Verification items for the finished model (mm, model axes). Round coordinates to 2 decimals unless told otherwise and drop trailing zeros. Write each loop counter-clockwise with the first axis right and the second up, starting at its lowest first coordinate (ties: lowest second). Pieces come first, ordered by that corner, then holes. Notation, with made-up numbers: (-10, 41) -> (15, 41) arc R20 cw to (15, 76) -> close; hole circle Ø6 at (25.25, -31). An arc over 180 degrees is marked (long way). Answer as a JSON object with one key per item and string values. Group by question number.
(1) Gauge pin test, flat end, axial feed: pin 1 Ø1.5 at (x, z) = (4.375, -5) entering from -Y. Record the tip position at first contact, or that the pin passes through.
(2) Scan lines: L1, parallel to X at y = 0.25, z = -168 (3 decimals); L2, parallel to X at y = 0.3, z = -37.5 (3 decimals); L3, parallel to Z at x = 3.5, y = 0.15. Record each from-to range of solid material in increasing order. Write a range as from..to.
(3) Sectioned sample at B-B on z = -103.5. Record the cut outline in (x, y) (3 decimals).
(4) Sectioned sample at A-A on y = 0.4. Count the separate pieces of the cut face and the enclosed holes in it, and give its area (3 significant figures).
```python
from build123d import *

# Parameters (mm, degrees)
SKETCH4_R           = 1.5
SKETCH4_R_2         = 1.25
BOSS_EXTRUDE2_DEPTH = 0.5


with BuildPart() as part:
    # Sketch4 → Boss-Extrude2 (new body)
    with BuildSketch(Plane(origin=(0, 0, 0), x_dir=(1, 0, 0), z_dir=(0, 1, 0))):
        with BuildLine():
            Line((0, 128.6), (0, 0))
            Line((0, 0), (-65.208953904, 0))
            ThreePointArc((-65.208953904, 0), (-75.225861161, 4.149138839), (-79.375, 14.166046096))
            Line((-79.375, 14.166046096), (-79.375, 50))
            Line((-79.375, 50), (-49.375, 50))
            Line((-49.375, 50), (-49.375, 118))
            Line((-49.375, 118), (-64.675, 118))
            ThreePointArc((-64.675, 118), (-75.069469683, 122.305530317), (-79.375, 132.7))
            Line((-79.375, 132.7), (-79.375, 193.786049975))
            add(Edge.make_bspline(
                [(-79.375, 193.786049975), (-78.783979858, 199.964089634), (-73.952599984, 211.643726286), (-54.660456042, 223.601842558), (-29.545703417, 228.182905558), (-9.188135392, 228.171492971), (0, 228.6)],
                knots=[0, 0, 0, 0, 0.226113446, 0.328670148, 0.719907193, 1, 1, 1, 1], degree=3))
            Line((0, 228.6), (0, 188.6))
            Line((0, 188.6), (-50, 188.6))
            ThreePointArc((-50, 188.6), (-51.25, 187.35), (-50, 186.1))
            Line((-50, 186.1), (0, 186.1))
            Line((0, 186.1), (0, 179.6))
            Line((0, 179.6), (-50, 179.6))
            ThreePointArc((-50, 179.6), (-51.25, 178.35), (-50, 177.1))
            Line((-50, 177.1), (0, 177.1))
            Line((0, 177.1), (0, 131.1))
            Line((0, 131.1), (-50, 131.1))
            ThreePointArc((-50, 131.1), (-51.25, 129.85), (-50, 128.6))
            Line((-50, 128.6), (0, 128.6))
        make_face()
        with Locations(Location((-74.875, 43, 0), (0, 0, 270))):
            Circle(SKETCH4_R, mode=Mode.SUBTRACT)
        with Locations(Location((-74.875, 18, 0), (0, 0, 270))):
            Circle(SKETCH4_R, mode=Mode.SUBTRACT)
        with Locations(Location((-39.375, 7.5, 0), (0, 0, 270))):
            Circle(SKETCH4_R, mode=Mode.SUBTRACT)
        with Locations(Location((-13.375, 7.5, 0), (0, 0, 270))):
            Circle(SKETCH4_R, mode=Mode.SUBTRACT)
        with Locations(Location((-4.375, 5, 0), (0, 0, 270))):
            Circle(SKETCH4_R_2, mode=Mode.SUBTRACT)
        with Locations(Location((-74.375, 143, 0), (0, 0, 270))):
            Circle(SKETCH4_R, mode=Mode.SUBTRACT)
        with Locations(Location((-74.375, 168, 0), (0, 0, 270))):
            Circle(SKETCH4_R, mode=Mode.SUBTRACT)
        with Locations(Location((-74.375, 193, 0), (0, 0, 270))):
            Circle(SKETCH4_R, mode=Mode.SUBTRACT)
        with Locations(Location((-39.375, 37.5, 0), (0, 0, 270))):
            Circle(SKETCH4_R, mode=Mode.SUBTRACT)
        with Locations(Location((-39.375, 67.5, 0), (0, 0, 270))):
            Circle(SKETCH4_R, mode=Mode.SUBTRACT)
        with Locations(Location((-12.875, 37.5, 0), (0, 0, 270))):
            Circle(SKETCH4_R, mode=Mode.SUBTRACT)
        with Locations(Location((-12.875, 67.5, 0), (0, 0, 270))):
            Circle(SKETCH4_R, mode=Mode.SUBTRACT)
    boss_extrude2 = extrude(amount=BOSS_EXTRUDE2_DEPTH)

    # Mirror4: part across plane


with BuildPart() as part_1:
    add(part.part)
    add(part.part.mirror(Plane(origin=(0, 0.5, -177.1), x_dir=(0, 0, 1), z_dir=(-1, 0, 0))))


with BuildPart() as mirror2_1:
    # Mirror2: Boss-Extrude2 across Right Plane
    add(boss_extrude2.mirror(Plane(origin=(0, 0, 0), x_dir=(0, 0, -1), z_dir=(1, 0, 0))))


with BuildPart() as part_2:
    add(part_1.part)

    # Mirror2 united with what the copies touc: union Mirror2_1
    add(mirror2_1.part)


solid = part_2.part
```
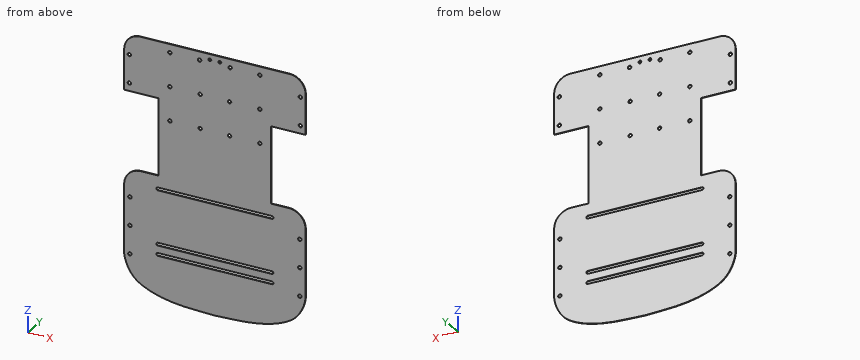
Computed values:
{
 "1": {"pin 1": "through"},
 "2": {"L1": "-79.375..-75.875, -72.875..72.875, 75.875..79.375", "L2": "-79.375..-40.875, -37.875..-14.375, -11.375..11.375, 14.375..37.875, 40.875..79.375", "L3": "-228.45..-188.6, -186.1..-179.6, -177.1..-131.1, -128.6..-5.89, -4.11..0"},
 "3": {"outline": "(-49.375, 0) -> (49.375, 0) -> (49.375, 0.5) -> (-49.375, 0.5) -> close"},
 "4": {"separate pieces": "1", "enclosed holes": "27", "area": "30,200 mm2"}
}
